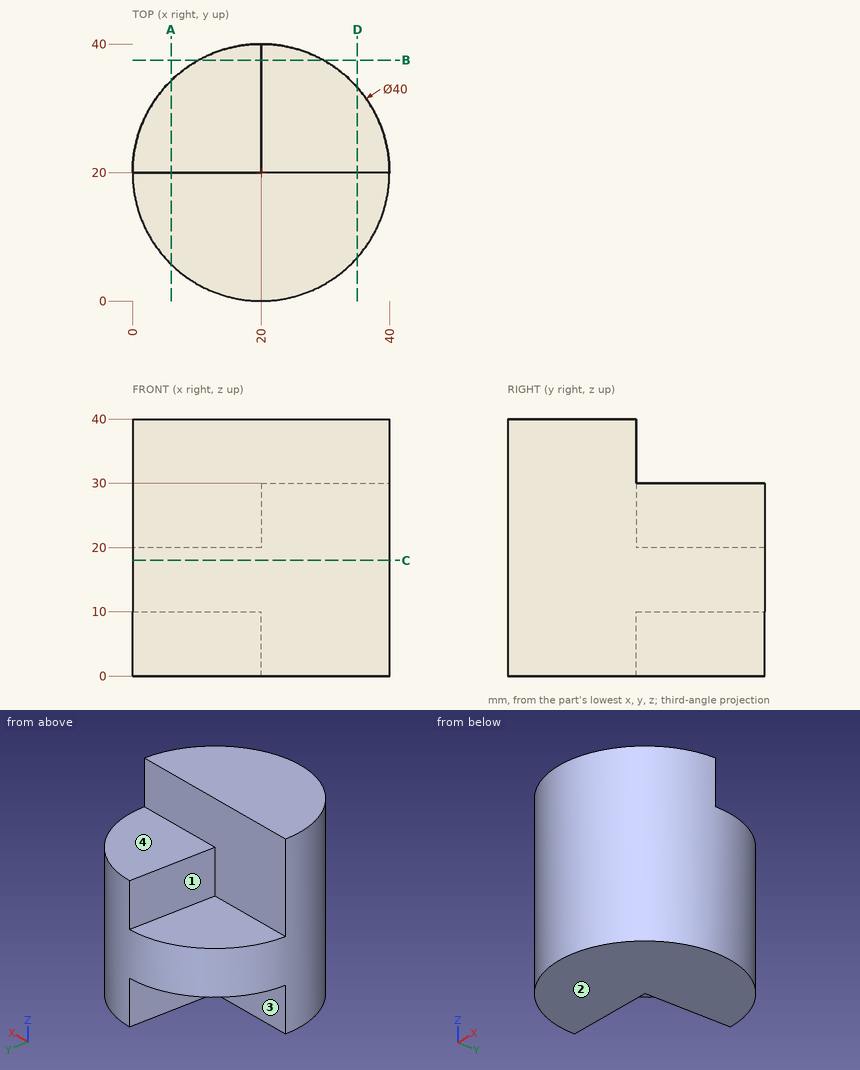
Geometry: see drawing. Coordinates: mm, zero at the bounding-box minimum. A direction names the side the tool comes from. Round coordinates to 2 decimals unless told otherwise and drop trailing zeros. Order: outer loops, then holes, each group sorted by start corner. A loop starts at its lowest first (then second) coordinate and runs counter-clockwise, first axis right, second up. Notation, with made-up numbers: (-31, 66.5) - (-16, 66.5) arc R30 cw to (-16, 97.5) - close; hole circle Ø2 at (63, 0.25). An arc over 180 degrees is marked (long way). Use a Markdown table: item, result. Add a question column.
1. Section query D-D (x = 35). Return the cut outline in (y, z), then the cut area to 3 significant figures.
2. Line query: probe 1 along Z at (x, y) = (19, 24.5); probe 2 along Z at (x, y) = (28, 38); probe 3 along Y at (x, z) = (6, 30). Output: solid intervals per line, ascending.
3. Section query C-C (z = 18). Return the cut outline in (x, y), then the cut area to 3 significant figures.
4. Section query A-A (x = 6). Return the cut outline in (y, z), then the cut area to 3 significant figures.
5. Set-up query: the marked faces 1, 2, 3 and 4. Return all of +Z, -Z, +X, -X, +Y, -Y with unobstructed straight access to the full face (end or side cutting, diameter ignored); none if empty.
6. First-contact query: pin 1 (3 mm diameter, centred on y = 6, z = 34.5, fed in from +X); pin 2 (22 mm diameter, centred on x = 31.5, y = 34.5, fed in from +Z); pin 3 (8 mm diameter, centred on y = 9, z = 34, fed in from -X) (3 decimals). Flat tips, straight axial feed; report the tip coordinate or a pass-through.
7. Section query B-B (y = 37.5). Return the cut outline in (x, z).
Derived:
| question | item | result |
|---|---|---|
| 1 | outline | (6.77, 0) - (33.23, 0) - (33.23, 30) - (20, 30) - (20, 40) - (6.77, 40) - close |
| 1 | area | 926 mm2 |
| 2 | probe 1 | 10 to 20 |
| 2 | probe 2 | 0 to 30 |
| 2 | probe 3 | 5.72 to 20 |
| 3 | outline | circle Ø40 at (20, 20) |
| 3 | area | 1,260 mm2 |
| 4 | outline | (5.72, 0) - (20, 0) - (20, 10) - (34.28, 10) - (34.28, 20) - (20, 20) - (20, 40) - (5.72, 40) - close |
| 4 | area | 714 mm2 |
| 5 | face 1 | +Z, -X, +Y |
| 5 | face 2 | -Z, +X, -X, +Y, -Y |
| 5 | face 3 | -Z, -X, +Y |
| 5 | face 4 | +Z, +X, -X, +Y |
| 6 | pin 1 | x = 35.61 |
| 6 | pin 2 | z = 30 |
| 6 | pin 3 | x = 1.265 |
| 7 | outline | (10.32, 10) - (20, 10) - (20, 0) - (29.68, 0) - (29.68, 30) - (20, 30) - (20, 20) - (10.32, 20) - close |
